Geometry: final body of the model. Coordinates: model frame, mm. Round coordinates to 2 decimals unless told otherwise and drop trailing zeros. Order: outer loops, then holes, each group sorted by start corner. A loop starts at its lowest first (then second) coordinate and runs counter-clockwise, first axis right, second up. Notation, with made-up numbers: M -22,-4.75 L 18,-4.75 A16 cw 18,22.25 Z; hole C -10.75,-26.75 d11. An arc over 180 degrees is marked long. Put each result on its own line as item: value. Start each with the question number.
1) Section C-C, the plane y = 12. Return loops of the section in (x, z), then the cut area to 3 significant figures.
2) Section B-B, the plane z = 1.5. Count the separate pieces of the cut face and the enclosed holes in it, then the cut area to 3 significant figures.
3) Section A-A, the plane x = 16. Return loops of the section in (y, z), then the cut area to 3 significant figures.
4) Draft query along X for faces 1 (the cylindrical face through (6.3, 4.1, 1)), 2 (the cylindrical face through (26.99, -17.15, 1.01)), 3 (the flat face through (0, 0, 0)). Return one class per face: pulls with the +X half, pulls with the -X half, needs draft (parallel to the pull), parting line crosses it, or undercut.
5) Material intervals for probe 1 along Y at (x, z) = (-7.5, 1.65); probe 2 along X at (y, z) = (5.5, 0.9); probe 3 along Y at (x, z) = (-8.5, 0.6), sorted ascending. Write a range as [from, to].
6) First-contact query: P1, Ø2.5, axis at x = -7.5, y = -13, coming from the -Z side; P2, Ø1, axis at y = 12.5, z = 1, coming from the +X side. Flat tips, straight axial feed; report the tip coordinate or a pass-through.
from build123d import *

# Parameters (mm, degrees)
SKETCH_1_W          = 60
SKETCH_1_H          = 40
SKETCH_1_R          = 1.25
EXTRUDE_1_DEPTH     = 2
FILLET_1_R          = 10
SKETCH_2_R          = 1.5
CUT_EXTRUDE_1_DEPTH = 2


with BuildPart() as part:
    # 草图1 → 凸台-拉伸1 (new body)
    with BuildSketch(Plane.XY):
        Rectangle(SKETCH_1_W, SKETCH_1_H)
        with Locations((-16, 12)):
            Circle(SKETCH_1_R, mode=Mode.SUBTRACT)
        with Locations((16, 12)):
            Circle(SKETCH_1_R, mode=Mode.SUBTRACT)
        with Locations((16, -12)):
            Circle(SKETCH_1_R, mode=Mode.SUBTRACT)
        with Locations((-16, -12)):
            Circle(SKETCH_1_R, mode=Mode.SUBTRACT)
    extrude(amount=EXTRUDE_1_DEPTH)

    # 圆角1
    fillet_1_edges = [part.edges().sort_by_distance(p)[0] for p in [
        (30, -20, 1),
        (-30, -20, 1),
        (-30, 20, 1),
        (30, 20, 1),
    ]]
    fillet(fillet_1_edges, radius=FILLET_1_R)

    # 草图2 → 切除-拉伸1 (cut)
    with BuildSketch(Plane.XY.offset(2)):
        with Locations((-7.5, 5)):
            Circle(SKETCH_2_R)
        with Locations((7.5, 5)):
            Circle(SKETCH_2_R)
        with Locations((7.5, -13)):
            Circle(SKETCH_2_R)
        with Locations((-7.5, -13)):
            Circle(SKETCH_2_R)
    extrude(amount=-CUT_EXTRUDE_1_DEPTH, mode=Mode.SUBTRACT)


solid = part.part
Result sheet:
1. outline: M -29.8,0 L -17.25,0 L -17.25,2 L -29.8,2 Z; M -14.75,0 L 14.75,0 L 14.75,2 L -14.75,2 Z; M 17.25,0 L 29.8,0 L 29.8,2 L 17.25,2 Z
1. area: 109 mm2
2. separate pieces: 1
2. enclosed holes: 8
2. area: 2,270 mm2
3. outline: M -20,0 L -13.25,0 L -13.25,2 L -20,2 Z; M -10.75,0 L 10.75,0 L 10.75,2 L -10.75,2 Z; M 13.25,0 L 20,0 L 20,2 L 13.25,2 Z
3. area: 70.0 mm2
4. face 1: undercut
4. face 2: pulls with the +X half
4. face 3: needs draft
5. probe 1: y = [-20, -14.5], [-11.5, 3.5], [6.5, 20]
5. probe 2: x = [-30, -8.91], [-6.09, 6.09], [8.91, 30]
5. probe 3: y = [-20, -14.12], [-11.88, 3.88], [6.12, 20]
6. P1: passes through
6. P2: stops at x = 29.8
